```python
from build123d import *

# Parameters (mm, degrees)
SKETCH_1_W          = 10
SKETCH_1_H          = 25
EXTRUDE_1_DEPTH     = 10
SKETCH_2_R          = 2.5
CUT_EXTRUDE_1_DEPTH = 10
CUT_EXTRUDE_2_REACH = 27
SKETCH_3_R          = 1.125
CUT_EXTRUDE_3_REACH = 27
SKETCH_4_R          = 1.125
SKETCH_5_W          = 10
SKETCH_5_H          = 25
EXTRUDE_2_DEPTH     = 2.5
SKETCH_6_W          = 10
SKETCH_6_H          = 40
EXTRUDE_3_DEPTH     = 3
SKETCH_7_R          = 1.4
CUT_EXTRUDE_4_DEPTH = 3


with BuildPart() as part:
    # 스케치1 → 보스-돌출1 (new body)
    with BuildSketch(Plane(origin=(0, 0, 0), x_dir=(1, 0, 0), z_dir=(0, 1, 0))):
        with Locations((-4.093959732, 10.604026846)):
            Rectangle(SKETCH_1_W, SKETCH_1_H)
    extrude(amount=EXTRUDE_1_DEPTH)

    # 스케치2 → 컷-돌출1 (cut)
    with BuildSketch(Plane.ZY.offset(9.093959732)):
        with Locations((-5.354026846, 5)):
            Circle(SKETCH_2_R)
        with Locations((-15.354026846, 5)):
            Circle(SKETCH_2_R)
    extrude(amount=-CUT_EXTRUDE_1_DEPTH, mode=Mode.SUBTRACT)

    # 스케치3 → 컷-돌출2 (cut, up to next)
    with BuildSketch(Plane.XY.offset(1.895973154), mode=Mode.PRIVATE) as cut_extrude_2_sk1:
        with Locations((-4.093959732, 5)):
            Circle(SKETCH_3_R)
    cut_extrude_2_tool1 = extrude(cut_extrude_2_sk1.sketch, amount=-CUT_EXTRUDE_2_REACH, mode=Mode.PRIVATE) & part.part
    add(cut_extrude_2_tool1.solids().sort_by_distance((-4.09396, 5, 1.895973))[0], mode=Mode.SUBTRACT)

    # 스케치4 → 컷-돌출3 (cut, up to next)
    with BuildSketch(Plane(origin=(0, 0, -23.104026846), x_dir=(-1, 0, 0), z_dir=(0, 0, -1)), mode=Mode.PRIVATE) as cut_extrude_3_sk1:
        with Locations((4.093959732, 5)):
            Circle(SKETCH_4_R)
    cut_extrude_3_tool1 = extrude(cut_extrude_3_sk1.sketch, amount=-CUT_EXTRUDE_3_REACH, mode=Mode.PRIVATE) & part.part
    add(cut_extrude_3_tool1.solids().sort_by_distance((-4.09396, 5, -23.104027))[0], mode=Mode.SUBTRACT)

    # 스케치5 → 보스-돌출2 (add)
    with BuildSketch(Plane.XZ):
        with Locations((-4.093959732, -10.604026846)):
            Rectangle(SKETCH_5_W, SKETCH_5_H)
    extrude(amount=EXTRUDE_2_DEPTH)

    # 스케치6 → 보스-돌출3 (add)
    with BuildSketch(Plane.XZ.offset(2.5)):
        with Locations((-4.093959732, -10.604026846)):
            Rectangle(SKETCH_6_W, SKETCH_6_H)
    extrude(amount=EXTRUDE_3_DEPTH)

    # 스케치7 → 컷-돌출4 (cut)
    with BuildSketch(Plane(origin=(0, -2.5, 0), x_dir=(1, 0, 0), z_dir=(0, 1, 0))):
        with Locations((-4.093959732, -5.645973154)):
            Circle(SKETCH_7_R)
        with Locations((-4.093959732, 26.854026846)):
            Circle(SKETCH_7_R)
    extrude(amount=-CUT_EXTRUDE_4_DEPTH, mode=Mode.SUBTRACT)


solid = part.part
```
Geometry check sheet. Reference: the model listing, model coordinates, mm. A direction names the side the tool comes from. Coordinates: 2 decimals unless noted, no trailing zeros. Order: outer loops, then holes, each group sorted by start corner. A loop starts at its lowest first (then second) coordinate and runs counter-clockwise, first axis right, second up.
Q1. Tool access check on faces 4 (the face through (-3.49, 5.95, -0.58)), 5 (the face through (-5, 4, 1.896)), 6 (the face through (-4.2, -2.5, -28.5)), 7 (the face through (-4.7, 5.95, -20.38)). Record the directions out of +Z, -Z, +X, -X, +Y, -Y that give a thin tool (end or side, any length) a straight path to the whole face; none if there is none.
Reply:
face 4: +Z
face 5: +Z, +X, -X, +Y
face 6: -Z, +X, -X, +Y
face 7: -Z
Q2. Sectioned sample at C-C on z = -6.5. Record the cut outline in (x, y), and give its area (3 significant figures).
Reply:
outline: (-9.09, -5.5) - (0.91, -5.5) - (0.91, 2.78) - (-9.09, 2.78) - close; (-9.09, 7.22) - (0.91, 7.22) - (0.91, 10) - (-9.09, 10) - close
area: 111 mm2
Q3. Sectioned sample at A-A on y = 5. Record the cut outline in (x, z).
Reply:
outline: (-9.09, -23.1) - (-5.22, -23.1) - (-5.22, -17.85) - (-9.09, -17.85) - close; (-9.09, -12.85) - (0.91, -12.85) - (0.91, -7.85) - (-9.09, -7.85) - close; (-9.09, -2.85) - (-5.22, -2.85) - (-5.22, 1.9) - (-9.09, 1.9) - close; (-2.97, -23.1) - (0.91, -23.1) - (0.91, -17.85) - (-2.97, -17.85) - close; (-2.97, -2.85) - (0.91, -2.85) - (0.91, 1.9) - (-2.97, 1.9) - close
Q4. Draft check along Z on faces 1 (the face through (0.906, 1, -11)), 2 (the face through (-4, -4, 9.396)), 3 (the face through (-4.16, 5.75, -12.97)). Enter one of: released by +Z, released by -Z, zero draft, split by the parting line, or undercut.
Reply:
face 1: zero draft
face 2: released by +Z
face 3: undercut
Q5. Sectioned sample at B-B on x = -6.75. Record the cut outline in (y, z).
Reply:
outline: (-5.5, -30.6) - (-2.5, -30.6) - (-2.5, -23.1) - (10, -23.1) - (10, 1.9) - (-2.5, 1.9) - (-2.5, 9.4) - (-5.5, 9.4) - close; hole circle Ø5 at (5, -15.35); hole circle Ø5 at (5, -5.35)
Q6. Thickness scan on probe 1 along X at (y, z) = (5, -21.75); probe 2 along Z at (x, y) = (-0.5, 4.5); probe 3 along Z at (x, y) = (-4.75, -4.75). Record the ranges inside material, lowest first.
Reply:
probe 1: x = -9.09 to -5.22, -2.97 to 0.91
probe 2: z = -23.1 to -17.8, -12.9 to -7.8, -2.9 to 1.9
probe 3: z = -30.6 to -28.09, -25.62 to 4.41, 6.88 to 9.4
Q7. Sectioned sample at D-D on x = -3.75. Record the cut outline in (y, z), and give its area (3 significant figures).
Reply:
outline: (-5.5, -30.6) - (-2.5, -30.6) - (-2.5, -28.21) - (-5.5, -28.21) - close; (-5.5, -25.5) - (-2.5, -25.5) - (-2.5, -23.1) - (3.93, -23.1) - (3.93, -17.61) arc R2.5 cw (long way) to (6.07, -17.61) - (6.07, -23.1) - (10, -23.1) - (10, 1.9) - (6.07, 1.9) - (6.07, -3.1) arc R2.5 cw (long way) to (3.93, -3.1) - (3.93, 1.9) - (-2.5, 1.9) - (-2.5, 4.29) - (-5.5, 4.29) - close; (-5.5, 7) - (-2.5, 7) - (-2.5, 9.4) - (-5.5, 9.4) - close
area: 355 mm2
Q8. Depth check by flat-ended pin: pin 1 Ø4 at (x, y) = (-6, 7.5) entering from +Z; pin 2 Ø6 at (x, y) = (-3.5, 4.5) entering from -Z; pin 3 Ø6 at (x, z) = (-5, 5.5) entering from +Y. Enter the tip coordinate at first touch or a pass-through.
Reply:
pin 1: stops at z = 1.9
pin 2: stops at z = -23.1
pin 3: stops at y = -2.5
